from build123d import *

# Parameters (mm, degrees)
SKETCH1_W                = 160
SKETCH1_H                = 98
BOSS_EXTRUDE1_DEPTH      = 39
M3_CLEARANCE_HOLE1_D     = 3.6
M3_CLEARANCE_HOLE1_DEPTH = 20
M3_CLEARANCE_HOLE1_TIP   = 1.081549114


with BuildPart() as part:
    # Sketch1 → Boss-Extrude1 (new body)
    with BuildSketch(Plane(origin=(0, 0, 0), x_dir=(1, 0, 0), z_dir=(0, 1, 0))):
        Rectangle(SKETCH1_W, SKETCH1_H)
    extrude(amount=BOSS_EXTRUDE1_DEPTH)

    # M3 Clearance Hole1
    with Locations(Plane(origin=(0, 0, 0), x_dir=(-1, 0, 0), z_dir=(0, -1, 0))):
        with Locations((-75, 44), (77, -43)):
            Hole(M3_CLEARANCE_HOLE1_D / 2, depth=M3_CLEARANCE_HOLE1_DEPTH)
            with Locations((0, 0, -(M3_CLEARANCE_HOLE1_DEPTH + M3_CLEARANCE_HOLE1_TIP / 2))):  # 118° drill point
                Cone(0, M3_CLEARANCE_HOLE1_D / 2, M3_CLEARANCE_HOLE1_TIP, mode=Mode.SUBTRACT)


solid = part.part
Can you work these out from the model? Positions are in its coordinate system, mm. A direction names the side the tool comes from. Round coordinates to 2 decimals unless told otherwise and drop trailing zeros. Answer in a Markdown table with one row per item. Add a question column.
Q1. We'd pull the mould along X, two halves only. Please class faces 1 (the cylindrical face through (73.673, 10.14, -45.217)), 2 (the flat face through (-1, 39, -1)), 3 (the flat face through (80, 19, 1)): pulls with the +X half, pulls with the -X half, needs draft (parallel to the pull), parting line crosses it, or undercut.
Q2. Which directions (+Z, -Z, +X, -X, +Y, -Y) give clear straight access to the entire face, cutting with the end or side of a thin tool? Please do faces 4 (the cylindrical face through (-78.327, 10.14, 41.783)), 5 (the flat face through (-1, 0, -1)).
Q3. I need wall thicknesses on L1, parallel to Z at x = 75, y = 5; L2, parallel to Z at x = -77, y = 11; L3, parallel to X at y = 5, z = -44. Which ranges of each line are inside material? Lowest first, please.
Q4. For pin 1 Ø3 at (x, z) = (75, -44) entering from -Y, with a flat end and sliding along its axis, tell me the tip position at first contact or that it passes through.
A:
| question | item | result |
|---|---|---|
| 1 | face 1 | undercut |
| 1 | face 2 | needs draft |
| 1 | face 3 | pulls with the +X half |
| 2 | face 4 | -Y |
| 2 | face 5 | +Z, -Z, +X, -X, -Y |
| 3 | L1 | -49 to -45.8, -42.2 to 49 |
| 3 | L2 | -49 to 41.2, 44.8 to 49 |
| 3 | L3 | -80 to 73.2, 76.8 to 80 |
| 4 | pin 1 | y = 20.18 |
